Here's how the part is built. I have some questions about the finished solid (model axes, mm). Face numbers are marked on the shaded views. A direction names the side the tool comes from. Round coordinates to 2 decimals unless told otherwise and drop trailing zeros. Loops run counter-clockwise (first coordinate to the right, second up) from the corner with the lowest first, then second, coordinate; pieces in that order, holes last. Notation, with made-up numbers: M 8.5,5.25 L 13.5,5.25 A15 cw 13.5,19.25 Z; hole C 9.25,80 d10. An arc over 180 degrees is marked long. Use a Markdown table: item, result.
from build123d import *

# Parameters (mm, degrees)
SKETCH1_W           = 60
SKETCH1_H           = 60
SKETCH1_R           = 3
BOSS_EXTRUDE1_DEPTH = 10
SKETCH2_W           = 66
SKETCH2_H           = 66
SKETCH2_W_2         = 60
SKETCH2_H_2         = 60
BOSS_EXTRUDE2_DEPTH = 2.5
CUT_EXTRUDE1_DEPTH  = 5
FILLET1_R           = 1


with BuildPart() as part:
    # Sketch1 → Boss-Extrude1 (new body)
    with BuildSketch(Plane(origin=(0, 0, 0), x_dir=(1, 0, 0), z_dir=(0, 1, 0))):
        Rectangle(SKETCH1_W, SKETCH1_H)
        with Locations(Location((0, 20.5, 0), (0, 0, 270))):
            Circle(SKETCH1_R, mode=Mode.SUBTRACT)
        with Locations(Location((20.5, 0, 0), (0, 0, 270))):
            Circle(SKETCH1_R, mode=Mode.SUBTRACT)
        with Locations(Location((0, -20.5, 0), (0, 0, 270))):
            Circle(SKETCH1_R, mode=Mode.SUBTRACT)
        with Locations(Location((-20.5, 0, 0), (0, 0, 270))):
            Circle(SKETCH1_R, mode=Mode.SUBTRACT)
    extrude(amount=BOSS_EXTRUDE1_DEPTH)

    # Sketch2 → Boss-Extrude2 (add)
    with BuildSketch(Plane(origin=(0, 10, 0), x_dir=(1, 0, 0), z_dir=(0, 1, 0))):
        Rectangle(SKETCH2_W, SKETCH2_H)
        Rectangle(SKETCH2_W_2, SKETCH2_H_2, mode=Mode.SUBTRACT)
    extrude(amount=-BOSS_EXTRUDE2_DEPTH)

    # Sketch3 → Cut-Extrude1 (cut)
    with BuildSketch(Plane(origin=(0, 10, 0), x_dir=(1, 0, 0), z_dir=(0, 1, 0))):
        Polygon((-4.734272207, 20.5), (-2.367136104, 16.4), (2.367136104, 16.4), (4.734272207, 20.5), (2.367136104, 24.6), (-2.367136104, 24.6), align=None)
        Polygon((-20.5, -4.734272207), (-16.4, -2.367136104), (-16.4, 2.367136104), (-20.5, 4.734272207), (-24.6, 2.367136104), (-24.6, -2.367136104), align=None)
        Polygon((20.5, 4.734272207), (16.4, 2.367136104), (16.4, -2.367136104), (20.5, -4.734272207), (24.6, -2.367136104), (24.6, 2.367136104), align=None)
        Polygon((4.734272207, -20.5), (2.367136104, -16.4), (-2.367136104, -16.4), (-4.734272207, -20.5), (-2.367136104, -24.6), (2.367136104, -24.6), align=None)
    extrude(amount=-CUT_EXTRUDE1_DEPTH, mode=Mode.SUBTRACT)

    # Fillet1
    fillet1_edges = [part.edges().sort_by_distance(p)[0] for p in [
        (33, 7.5, 0),
        (33, 8.75, -33),
        (0, 7.5, 33),
        (33, 8.75, 33),
        (-33, 7.5, 0),
        (-33, 8.75, 33),
        (0, 7.5, -33),
        (-33, 8.75, -33),
        (33, 10, 0),
        (0, 10, -33),
        (-33, 10, 0),
        (0, 10, 33),
    ]]
    fillet(fillet1_edges, radius=FILLET1_R)


solid = part.part
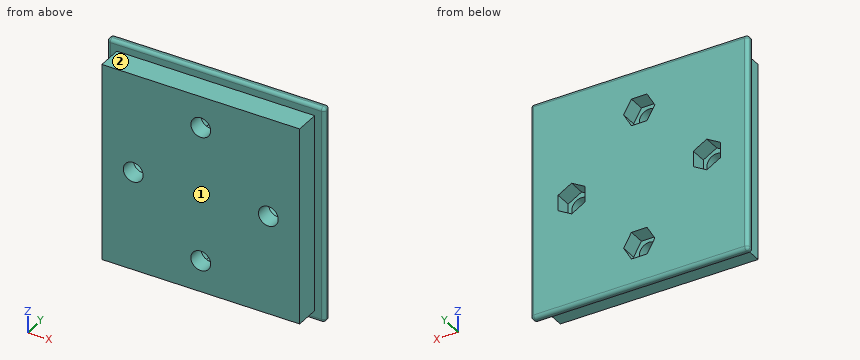
1. Imagine slicing it at D-D, the plane z = 11. Write out the boundary of the cut face in (x, y), then the cut area to 3 significant figures.
Answer sheet:
| item | result |
|---|---|
| outline | M -33,8.5 A1 ccw -32,7.5 L -30,7.5 L -30,0 L 30,0 L 30,7.5 L 32,7.5 A1 ccw 33,8.5 L 33,9 A1 ccw 32,10 L -32,10 A1 ccw -33,9 Z |
| area | 614 mm2 |
2. Imagine slicing it at C-C, the plane x = -26. Write out the boundary of the cut face in (y, z), then the cut area to 3 significant figures.
Answer sheet:
| item | result |
|---|---|
| outline | M 0,-30 L 7.5,-30 L 7.5,-32 A1 ccw 8.5,-33 L 9,-33 A1 ccw 10,-32 L 10,32 A1 ccw 9,33 L 8.5,33 A1 ccw 7.5,32 L 7.5,30 L 0,30 Z |
| area | 614 mm2 |
3. Imagine slicing it at A-A, the plane x = 0. Write out the boundary of the cut face in (y, z).
Answer sheet:
| item | result |
|---|---|
| outline | M 0,-30 L 7.5,-30 L 7.5,-32 A1 ccw 8.5,-33 L 9,-33 A1 ccw 10,-32 L 10,-24.6 L 5,-24.6 L 5,-23.5 L 0,-23.5 Z; M 0,-17.5 L 5,-17.5 L 5,-16.4 L 10,-16.4 L 10,16.4 L 5,16.4 L 5,17.5 L 0,17.5 Z; M 0,23.5 L 5,23.5 L 5,24.6 L 10,24.6 L 10,32 A1 ccw 9,33 L 8.5,33 A1 ccw 7.5,32 L 7.5,30 L 0,30 Z |
4. I need wall thicknesses on probe 1 along Z at (x, y) = (0, 3.6); probe 2 along X at (y, z) = (3.5, 27). Which ranges of each line are inside material? Lowest first, please. Write a range as from..to.
Answer sheet:
| item | result |
|---|---|
| probe 1 | -30..-23.5, -17.5..17.5, 23.5..30 |
| probe 2 | -30..30 |
5. Which directions (+Z, -Z, +X, -X, +Y, -Y) give clear straight access to the entire face, cutting with the end or side of a thin tool? Please do the marked faces 1 and 2.
Answer sheet:
| item | result |
|---|---|
| face 1 | +Z, -Z, +X, -X, -Y |
| face 2 | +Z, +X, -X, -Y |
6. For pin 1 Ø1 at (y, z) = (1.5, -10) entering from -X; pin 2 Ø1.4 at (y, z) = (7.5, -0.5) entering from +X; pin 3 Ø6.5 at (x, z) = (21, 0) entering from +Y; pin 4 Ø5.5 at (x, z) = (20.5, 0) entering from -Y, each with a flat end and sliding along its axis, tell me the tip position at first contact or that it passes through.
Answer sheet:
| item | result |
|---|---|
| pin 1 | x = -30 |
| pin 2 | x = 32.95 |
| pin 3 | y = 5 |
| pin 4 | through |
7. Imagine slicing it at B-B, the plane y = 2.75. Write out the boundary of the cut face in (x, z).
Answer sheet:
| item | result |
|---|---|
| outline | M -30,-30 L 30,-30 L 30,30 L -30,30 Z; hole C -20.5,0 d6; hole C 0,-20.5 d6; hole C 0,20.5 d6; hole C 20.5,0 d6 |
